Can you work these out from the model? Positions are in its coordinate system, mm. Face numbers are marked on the shaded views. A direction names the side the tool comes from. Give positions to 0.01 mm unless a question says otherwise; leave off trailing zeros. Loops run counter-clockwise (first coordinate to the right, second up) from the corner with the lowest first, then second, coordinate; pieces in that order, holes last. Notation, with made-up numbers: (62, 52) -> (77, 52) arc R24 cw to (77, 66) -> close; hole circle Ø8 at (38, 54). An arc over 180 degrees is marked (long way). Return JSON: item names as keys, results as strings. Group by question number.
Q1. Suppose I cut it at B-B, the plane y = 0.5. Please give me the cut outline in (x, z).
Q2. Suppose I cut it at A-A, the plane x = 0. Please give me the cut outline in (y, z), and give its area (3 significant figures).
Q3. Will these pins go through, and if not, where does the flat tip stop? pin 1 (1.5 mm diameter, centred on x = -0.5, z = -1, fed in from +Y); pin 2 (0.5 mm diameter, centred on x = -1, z = 2.5, fed in from -Y); pin 3 (1.6 mm diameter, centred on x = 0.5, y = 0, fed in from +Z).
Q4. Thinking about a two-plate mould opening in Y: for the marked faces 3, 4, 5 and 6, which applies, pulls with the +Y half, pulls with the -Y half, needs draft (parallel to the pull), parting line crosses it, or undercut?
Q5. Which directions (+Z, -Z, +X, -X, +Y, -Y) give clear straight access to the entire face, cutting with the end or side of a thin tool? Please do the marked faces 1 and 2.
Q6. I need wall thicknesses on line 1 along Z through (x, y) = (1.5, 0); line 2 along Z through (x, y) = (2.5, -0.25); line 3 along X through (y, z) = (-2.75, 1.75). Which ranges of each line are inside material? Lowest first, please. Write a range as [from, to].
Q7. Suppose I cut it at D-D, the plane z = -3.25. Please give me the cut outline in (x, y), and give its area (3 significant figures).
Q8. Suppose I cut it at C-C, the plane z = 1.5. Please give me the cut outline in (x, y).
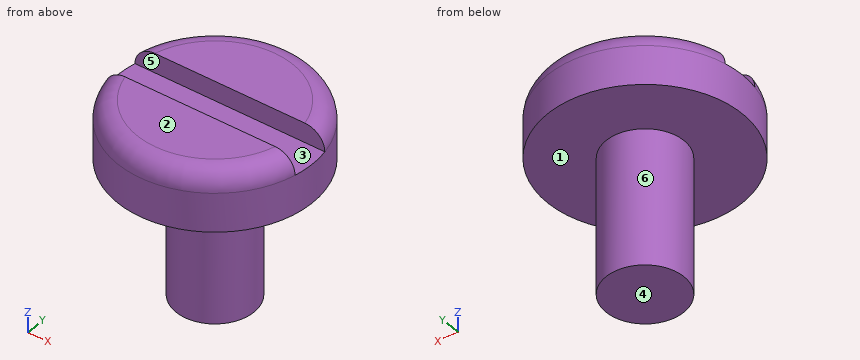
Autodesk Inventor part; units mm, degrees
ref_plane "YZ Plane" through (0, 0, 0) normal (1, 0, 0) x (0, 1, 0)
ref_plane "XZ Plane" through (0, 0, 0) normal (0, 1, 0) x (-1, 0, 0)
ref_plane "XY Plane" through (0, 0, 0) normal (0, 0, 1) x (1, 0, 0)
sketch "Sketch1" plane through (0, 0, 0) normal (0, 0, 1) x (1, 0, 0)
  circle A0 centre (0, 0) radius 5
  dimension "d0" = 10
extrude "Extrusion1" add sketch "Sketch1" along normal blind 3
sketch "Sketch2" plane through (0, 0, 3) normal (0, 0, 1) x (1, 0, 0)
  circle A0 centre (0, 0) radius 5
  line L0 (-4.899, 1) -> (4.899, 1)
  line L1 (7.3763, 1) -> (7.3763, -1)
  line L2 (4.899, -1) -> (-4.899, -1)
  line L3 (-7.3763, -1) -> (-7.3763, 1)
  line L4 (-7.3763, 1) -> (7.3763, -1) construction
  line L5 (7.3763, 1) -> (-7.3763, -1) construction
  circle A1 centre (0, 0) radius 5
  dimension "d3" = 2
  dimension "d4" = 82.28
  dimension "d5" = 82.28
  dimension "d6" = 2
  dimension "d7" = 1
extrude "Extrusion2" cut sketch "Sketch2" against normal blind 1 contours A0 L2 L0
fillet "Fillet1" radius 1 2 edges at (0, 5, 3) (0, -5, 3)
sketch "Sketch3" plane through (0, 0, 0) normal (0, 0, -1) x (-1, 0, 0)
  circle A0 centre (0, 0) radius 5
  circle A1 centre (0, 0) radius 2
  dimension "d11" = 4
extrude "Extrusion3" add sketch "Sketch3" along normal blind 7 contours A1
thread "Thread1"
properties part number "17A - Crosshead pin1" material "Steel AISI 1020 107 HR"
Ans:
{
 "1": {"outline": "(-4.97, 0) -> (-1.94, 0) -> (-1.94, -7) -> (1.94, -7) -> (1.94, 0) -> (4.97, 0) -> (4.97, 2) -> (-4.97, 2) -> close"},
 "2": {"outline": "(-5, 0) -> (-2, 0) -> (-2, -7) -> (2, -7) -> (2, 0) -> (5, 0) -> (5, 2) arc R1 ccw to (4, 3) -> (1, 3) -> (1, 2) -> (-1, 2) -> (-1, 3) -> (-4, 3) arc R1 ccw to (-5, 2) -> close", "area": "55.6 mm^2"},
 "3": {"pin 1": "stops at y = 2", "pin 2": "stops at y = -4.88", "pin 3": "stops at z = 2"},
 "4": {"face 3": "undercut", "face 4": "needs draft", "face 5": "undercut", "face 6": "parting line crosses it"},
 "5": {"face 1": "-Z", "face 2": "+Z, +X, -X, +Y, -Y"},
 "6": {"line 1": "z = [-7, 2]", "line 2": "z = [0, 2]", "line 3": "x = [-4.18, 4.18]"},
 "7": {"outline": "circle Ø4 at (0, 0)", "area": "12.6 mm^2"},
 "8": {"outline": "circle Ø10 at (0, 0)"}
}
